Can you work these out from the model? Positions are in its coordinate system, mm. A direction names the side the tool comes from. Give positions to 0.01 mm unless a question says otherwise; leave off trailing zeros. Order: outer loops, then holes, each group sorted by start corner. A loop starts at its lowest first (then second) coordinate and runs counter-clockwise, first axis right, second up. Notation, with made-up numbers: (19, 5.5) - (40, 5.5) arc R12 ccw to (40, 20.5) - close; hole circle Ø8 at (30, 23.5). An arc over 180 degrees is marked (long way). Answer as a JSON object with one key per item and string values.
```python
from build123d import *

# Parameters (mm, degrees)
SKETCH1_R           = 1.5
BOSS_EXTRUDE1_DEPTH = 2


with BuildPart() as part:
    # Sketch1 → Boss-Extrude1 (new body)
    with BuildSketch(Plane.XY):
        with BuildLine():
            Line((0, 0), (0, 18.000341084))
            Line((0, 18.000341084), (4, 18.000341084))
            Line((4, 18.000341084), (4, 14.000341084))
            Line((4, 14.000341084), (9.631516349, 14.000341084))
            Line((9.631516349, 14.000341084), (9.631516349, 18.000341084))
            Line((9.631516349, 18.000341084), (30.123176491, 13.320805491))
            ThreePointArc((30.123176491, 13.320805491), (35.324106187, 5.989458303), (28.621516349, 0))
            Line((28.621516349, 0), (9.631516349, 0))
            Line((9.631516349, 0), (9.631516349, 4))
            Line((9.631516349, 4), (4, 4))
            Line((4, 4), (4, 0))
            Line((4, 0), (0, 0))
        make_face()
        with Locations((28.621516349, 6.745044143)):
            Circle(SKETCH1_R, mode=Mode.SUBTRACT)
        Polygon((14.250450019, 12.02557168), (12.280834513, 11.678275325), (13.149075402, 6.75423656), (15.118690908, 7.101532915), align=None, mode=Mode.SUBTRACT)
        Polygon((7.356795748, 10.810034437), (8.225036637, 5.885995672), (6.255421131, 5.538699316), (5.387180242, 10.462738081), align=None, mode=Mode.SUBTRACT)
    extrude(amount=BOSS_EXTRUDE1_DEPTH)


solid = part.part
```
Q1. I need wall thicknesses on L1, parallel to X at y = 6.5, z = 1; L2, parallel to X at y = 10, z = 1.7; L3, parallel to Y at x = 8.5, z = 1.85. Which ranges of each line are inside material? Lowest first, please.
Recorded:
{"L1": "x = 0 to 6.09, 8.12 to 27.14, 30.1 to 35.36", "L2": "x = 0 to 5.47, 7.5 to 12.58, 14.61 to 34.53", "L3": "y = 4 to 14"}
Q2. If we section it at A-A, the plane y = 6.25: Please give me the cut outline in (x, z).
Recorded:
{"outline": "(0, 0) - (6.13, 0) - (6.13, 2) - (0, 2) - close; (8.16, 0) - (27.21, 0) - (27.21, 2) - (8.16, 2) - close; (30.04, 0) - (35.35, 0) - (35.35, 2) - (30.04, 2) - close"}
Q3. I'm going to push flat-ended pins straight in: pin 1 Ø0.6 at (x, z) = (6.5, 1) entering from -Y; pin 2 Ø1 at (x, z) = (8, 0.5) entering from +Y. Where does each tip first touch, or does it pass through?
Recorded:
{"pin 1": "stops at y = 4", "pin 2": "stops at y = 14"}
Q4. We'd pull the mould along Y, two halves only. Please class faces 4 (the face through (6.358, 10.634, 0.986)), 5 (the face through (4, 16, 1)), 6 (the face through (5.827, 7.966, 0.986)), 7 (the face through (7, 14, 1)): released by +Y, released by -Y, zero draft, split by the parting line, or undercut.
Recorded:
{"face 4": "undercut", "face 5": "zero draft", "face 6": "undercut", "face 7": "released by +Y"}
Q5. If we section it at B-B, the plane x = 28: Please give me the cut outline in (y, z).
Recorded:
{"outline": "(0, 0) - (5.38, 0) - (5.38, 2) - (0, 2) - close; (8.11, 0) - (13.81, 0) - (13.81, 2) - (8.11, 2) - close"}
Q6. If we section it at D-D, the plane y = 2.75: Please give me the cut outline in (x, z).
Recorded:
{"outline": "(0, 0) - (4, 0) - (4, 2) - (0, 2) - close; (9.63, 0) - (34.06, 0) - (34.06, 2) - (9.63, 2) - close"}
Q7. Which directions (+Z, -Z, +X, -X, +Y, -Y) give clear straight access to the entire face, cutting with the end or side of a thin tool? Please do faces 1 (the face through (7.785, 8.382, 0.986)), 2 (the face through (35.34, 6.13, 0.99)), 3 (the face through (4, 2, 1)).
Recorded:
{"face 1": "+Z, -Z", "face 2": "+Z, -Z, +X", "face 3": "+Z, -Z, -Y"}
Q8. If we section it at C-C, the plane z = 0.35: Please give me the cut outline in (x, y).
Recorded:
{"outline": "(0, 0) - (4, 0) - (4, 4) - (9.63, 4) - (9.63, 0) - (28.62, 0) arc R6.75 ccw to (30.12, 13.32) - (9.63, 18) - (9.63, 14) - (4, 14) - (4, 18) - (0, 18) - close; hole (5.39, 10.46) - (6.26, 5.54) - (8.23, 5.89) - (7.36, 10.81) - close; hole (12.28, 11.68) - (13.15, 6.75) - (15.12, 7.1) - (14.25, 12.03) - close; hole circle Ø3 at (28.62, 6.75)"}
